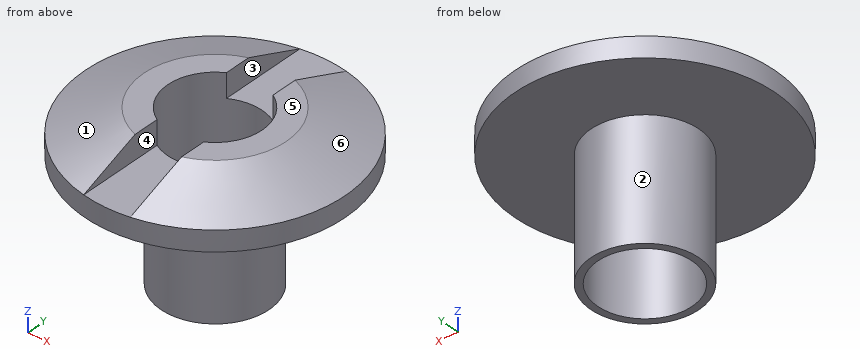
```python
from build123d import *

# Parameters (mm, degrees)
F2_W     = 1.8542
F2_H     = 0.9525
F3_DEPTH = 6.35
F4_R     = 1.8796
F5_DEPTH = 6.5288


with BuildPart() as f1:
    # F0 (on Front) → F1 (revolve)
    with BuildSketch(Plane.XZ):
        Polygon((17.789439, 2.350953), (17.789439, 8.878753), (14.957339, 8.878753), (12.607839, 7.926253), (12.607839, 7.113453), (15.635291, 7.113453), (15.635291, 2.350953), align=None)
    revolve(axis=Axis((17.789439, 0, 5.614853), (0, 0, -1)))

    # F2 (on Front) → F3 (cut, symmetric)
    with BuildSketch(Plane.XZ):
        with Locations((17.789439, 8.402503)):
            Rectangle(F2_W, F2_H)
    extrude(amount=F3_DEPTH, both=True, mode=Mode.SUBTRACT)

    # F4 (on face) → F5 (cut, through all)
    with BuildSketch(Plane(origin=(0, 0, 2.350953), x_dir=(1, 0, 0), z_dir=(0, 0, -1))):
        with Locations((17.789439, 0)):
            Circle(F4_R)
    extrude(amount=-F5_DEPTH, mode=Mode.SUBTRACT)


solid = f1.part
```
Check sheet for the modelled part. Datum: model origin and axes. Units: mm. Face numbers are marked on the shaded views. A direction names the side the tool comes from. Give positions to 0.01 mm unless a question says otherwise; leave off trailing zeros. Order: outer loops, then holes, each group sorted by start corner. A loop starts at its lowest first (then second) coordinate and runs counter-clockwise, first axis right, second up. Notation, with made-up numbers: (35.25, -37.75) -> (60.25, -37.75) arc R14 cw to (60.25, -33.75) -> close; hole circle Ø3 at (-5, 67). An arc over 180 degrees is marked (long way). Use CSV: the item, a comma, the result in double quotes. Start each with the question number.
1) Sectioned sample at A-A, the plane y = 0. Record the boundary of the cut face in (x, z).
2) Sectioned sample at D-D, the plane z = 8.25. Record the boundary of the cut face in (x, y), plus the area to 3 significant figures.
3) Sectioned sample at C-C, the plane z = 3. Record the boundary of the cut face in (x, y), plus the area to 3 significant figures.
4) Set-up check for the marked faces 1, 2 and 3: record each of +Z, -Z, +X, -X, +Y, -Y from which the full face is reachable in a straight line by a thin tool's end or side.
5) Mould release check, pull along X, two halves, no side actions. Record for the marked faces 4, 5 and 6: released by +X, released by -X, zero draft, split by the parting line, or undercut.
6) Material ranges on line 1 (X direction, y = 0, z = 7.25); line 2 (Z direction, x = 17.5, y = 2.25); line 3 (Y direction, x = 17.75, z = 5.25), recorded low to high. Write a range as from..to.
7) Go/stop test with flat-tipped pins: P1, Ø0.9, axis at x = 17.5, y = 3.5, coming from the +Z side; P2, Ø1, axis at y = 2.5, z = 8, coming from the -X side; P3, Ø2, axis at x = 15, z = 4.5, coming from the +Y side. Record where each tip stops, or that it passes through.
8) Sectioned sample at B-B, the plane x = 17.5. Record the boundary of the cut face in (y, z), plus the area to 3 significant figures.
Recorded:
1,outline,"(12.61, 7.11) -> (15.64, 7.11) -> (15.64, 2.35) -> (15.91, 2.35) -> (15.91, 8.88) -> (14.96, 8.88) -> (12.61, 7.93) -> close; (19.67, 2.35) -> (19.94, 2.35) -> (19.94, 7.11) -> (22.97, 7.11) -> (22.97, 7.93) -> (20.62, 8.88) -> (19.67, 8.88) -> close"
2,outline,"(16.86, -4.28) -> (16.86, -1.64) arc R1.88 cw to (16.86, 1.64) -> (16.86, 4.28) arc R4.38 ccw to start; (18.72, -4.28) arc R4.38 ccw to (18.72, 4.28) -> (18.72, 1.64) arc R1.88 cw to (18.72, -1.64) -> close"
2,area,"39.8 mm2"
3,outline,"circle Ø4.31 at (17.79, 0); hole circle Ø3.76 at (17.79, 0)"
3,area,"3.48 mm2"
4,face 1,"+Z, -X"
4,face 2,"-Z"
4,face 3,"+Z, +Y, -Y"
5,face 4,"undercut"
5,face 5,"zero draft"
5,face 6,"released by +X"
6,line 1,"12.61..15.91, 19.67..22.97"
6,line 2,"7.11..7.93"
6,line 3,"-2.15..-1.88, 1.88..2.15"
7,P1,"z = 7.93"
7,P2,"x = 13.01"
7,P3,"y = 1.2"
8,outline,"(-5.17, 7.11) -> (-2.13, 7.11) -> (-2.13, 2.35) -> (-1.86, 2.35) -> (-1.86, 7.93) -> (-5.17, 7.93) -> close; (1.86, 2.35) -> (2.13, 2.35) -> (2.13, 7.11) -> (5.17, 7.11) -> (5.17, 7.93) -> (1.86, 7.93) -> close"
8,area,"8.03 mm2"
